from build123d import *

# Parameters (mm, degrees)
SKETCH_1_R      = 0.999998023
SKETCH_1_R_2    = 1.000000976
EXTRUDE_1_DEPTH = 2.000000328


with BuildPart() as part:
    # Эскиз1 → Бобышка-Вытянуть1 (new body)
    with BuildSketch(Plane.XZ.offset(23.000000045)):
        Polygon((-84.028117359, -2.202427713), (-83.852753043, -2.287971787), (-83.6712569, -2.35957955), (-83.484724164, -2.416815143), (-83.294294775, -2.45932932), (-83.101138473, -2.486863639), (-82.906417549, -2.499250229), (-82.711324096, -2.496413421), (-82.517042756, -2.478370909), (-82.324765623, -2.445232356), (-82.135654986, -2.397199627), (-81.950873137, -2.334565157), (-81.771530211, -2.257710788), (-81.598728895, -2.167104278), (-81.433527172, -2.063297899), (-81.276915967, -1.946923556), (-81.129856408, -1.818690565), (-80.993250012, -1.679379493), (-80.867916346, -1.529839239), (-80.754637718, -1.370980637), (-80.654084682, -1.203771099), (-80.566875637, -1.029229374), (-80.493554473, -0.848418393), (-80.434553325, -0.662439677), (-80.390237272, -0.472426036), (-80.360867083, -0.279534725), (-80.346636474, -0.084940737), (-80.347619951, 0.110170622), (-80.363817513, 0.304610934), (-80.395124853, 0.497195811), (-80.441370606, 0.686752202), (-80.50224185, 0.872125558), (-80.577395856, 1.052186592), (-80.666355789, 1.225838787), (-80.768592656, 1.392024336), (-80.883473158, 1.549730659), (-81.010304391, 1.697997563), (-81.148318946, 1.835921779), (-81.296652555, 1.96266314), (-81.454440951, 2.077449812), (-81.620678306, 2.17958237), (-81.794388592, 2.268439159), (-81.974491477, 2.343478147), (-82.159906626, 2.40424322), (-82.349486649, 2.450363711), (-82.542091608, 2.481558593), (-82.736544311, 2.49763811), (-82.931652665, 2.49850424), (-83.126246929, 2.484151861), (-83.319112659, 2.454668051), (-83.509102464, 2.410232788), (-89.923687279, 7.373288274), (-110.284693539, 12.718074955), (-110.365286469, 12.895765714), (-110.459499061, 13.066628017), (-110.566742718, 13.229624368), (-110.68636924, 13.383760117), (-110.817655921, 13.528098352), (-110.959798098, 13.66175618), (-111.111931503, 13.78392335), (-111.273132265, 13.893852942), (-111.442416906, 13.990878128), (-111.618742347, 14.074404724), (-111.801050603, 14.143927023), (-111.98823154, 14.199018478), (-112.179122865, 14.239346609), (-112.372592092, 14.264663681), (-112.567447126, 14.274815097), (-112.762488425, 14.269742183), (-112.956546247, 14.249472879), (-113.1484285, 14.214130118), (-113.336972892, 14.163931832), (-113.521032035, 14.099182561), (-113.699480891, 14.020276256), (-113.871231675, 13.927693479), (-114.035241306, 13.821999542), (-114.190496504, 13.703836128), (-114.336073399, 13.573925011), (-114.471077919, 13.433056884), (-114.594690502, 13.282089494), (-114.706136286, 13.121941127), (-114.804767072, 12.95358967), (-114.889964461, 12.778058648), (-114.961214364, 12.596419081), (-115.018077195, 12.409775518), (-115.060210228, 12.219266966), (-115.087367594, 12.026051059), (-115.099363029, 11.831306852), (-115.096144378, 11.636218987), (-115.077711642, 11.441977695), (-115.04419893, 11.249764822), (-114.995785058, 11.060751043), (-114.932790399, 10.876088403), (-114.855580032, 10.696900077), (-114.764630795, 10.524280369), (-114.66050148, 10.35927888), (-114.543817937, 10.202899575), (-114.415287971, 10.05609706), (-114.275708795, 9.919765405), (-114.125922322, 9.794733487), (-113.966837525, 9.681764059), (-113.79943043, 9.581544437), (-113.624714315, 9.494686499), (-113.443754613, 9.421717376), (-113.257668912, 9.363083169), (-113.067567348, 9.319140576), (-112.874612212, 9.290155955), (-112.679995596, 9.276308119), (-112.484887242, 9.277679026), (-112.290471792, 9.294263087), (-112.09795624, 9.325955994), (-111.908487976, 9.372567758), (-111.72323674, 9.433813393), (-111.54332757, 9.50931944), (-111.369848251, 9.598624893), (-111.203864217, 9.701187722), (-111.046388745, 9.816383012), (-91.276302934, 4.62671183), (-85.344910622, 0.037510123), (-85.340216756, -0.157547402), (-85.320338607, -0.351645285), (-85.285380483, -0.543601287), (-85.235551, -0.732246088), (-85.171163082, -0.916430785), (-85.092611611, -1.095033367), (-85.000365973, -1.266965992), (-84.894999862, -1.431181328), (-84.777146578, -1.586679369), (-84.647521377, -1.73251261), (-84.50692147, -1.867792918), (-84.356203675, -1.991696423), (-84.196276963, -2.10346817), align=None)
        with Locations(Location((-82.845189618, -1.945e-06, 0), (0, 0, 270))):
            Circle(SKETCH_1_R, mode=Mode.SUBTRACT)
        with Locations(Location((-112.600002971, 11.775028493, 0), (0, 0, 270))):
            Circle(SKETCH_1_R_2, mode=Mode.SUBTRACT)
    extrude(amount=-EXTRUDE_1_DEPTH)


solid = part.part
Geometry: final body of the model. Coordinates: model frame, mm. Give positions to 0.01 mm unless a question says otherwise; leave off trailing zeros. Write each loop counter-clockwise with the first axis right and the second up, starting at its lowest first coordinate (ties: lowest second). Pieces come first, ordered by that corner, then holes. Notation, with made-up numbers: (-35, -5.5) - (-10, -5.5) arc R30 ccw to (-10, 33.5) - close; hole circle Ø11 at (57, 28.5). An arc over 180 degrees is marked (long way). Return JSON: item names as keys, results as strings. Group by question number.
1) Section C-C on z = 6.5. Return the cut outline in (x, y) (3 decimals), plus the area to 3 significant figures.
2) Mould query, pull axis Z, two halves, no side actions, for faces 1 (the cylindrical face through (-113.576, -22.014, 11.992)), 2 (the flat face through (-88.4, -22, 2.4)), 3 (the flat face through (-86.671, -22.014, 4.857)). Classes: released by +Z, released by -Z, zero draft, split by the parting line, or undercut.
3) First-contact query: P1, Ø4, axis at x = -88, z = 2, coming from the +Y side. Flat tip, straight axial feed; report the tip coordinate or a pass-through.
4) Section B-B on x = -104. Return the cut outline in (y, z), plus the area to 3 significant figures.
5) Section A-A on y = -22.25. State how many separate pieces and enclosed holes the cut face has, plus the area to 3 significant figures.
6) Line query: line 1 (Z direction, x = -113, y = -22.9); line 2 (Z direction, x = -83, y = -21.45); line 3 (Z direction, x = -102.5, y = -22.35). Output: solid intervals per line, ascending.
Filled in:
{
 "1": {"outline": "(-98.413, -23) - (-88.795, -23) - (-88.795, -21) - (-98.413, -21) - close", "area": "19.2 mm^2"},
 "2": {"face 1": "undercut", "face 2": "released by -Z", "face 3": "released by +Z"},
 "3": {"P1": "stops at y = -21"},
 "4": {"outline": "(-23, 7.97) - (-21, 7.97) - (-21, 11.07) - (-23, 11.07) - close", "area": "6.20 mm^2"},
 "5": {"separate pieces": "1", "enclosed holes": "2", "area": "117 mm^2"},
 "6": {"line 1": "z = 9.31 to 10.86, 12.69 to 14.24", "line 2": "z = -2.49 to -0.99, 0.99 to 2.49", "line 3": "z = 7.57 to 10.67"}
}
